Design review of the part shown in the three views and the two pictorial views. Dimensions are in mm from the part's minimum x, y and z. Give positions to 0.01 mm unless a question says otherwise; leave off trailing zeros. Order: outer loops, then holes, each group sorted by start corner. A loop starts at its lowest first (then second) coordinate and runs counter-clockwise, first axis right, second up.
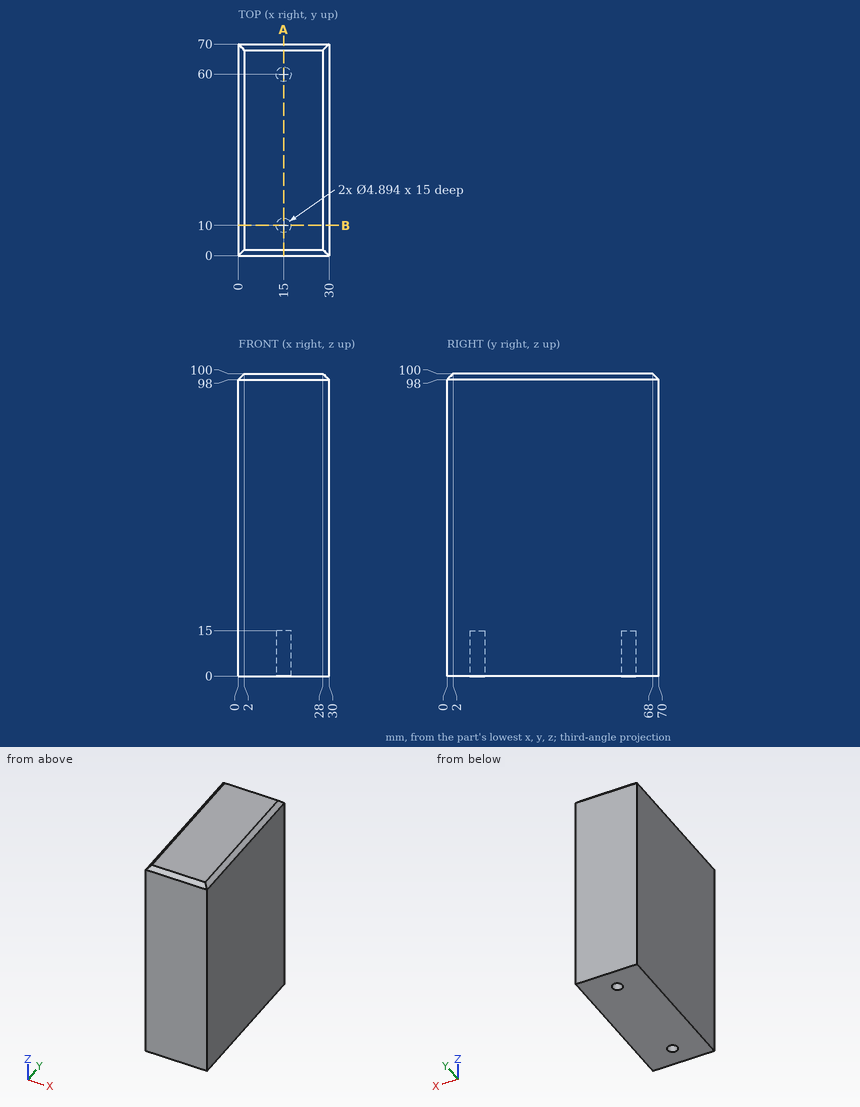
Item 1: For line 1 (Y direction, x = 15, z = 10); line 2 (X direction, y = 10, z = 7.25), list the stretches that pass through material, from the lowest coordinate up.
Values found:
line 1: y = 0 to 7.55, 12.45 to 57.55, 62.45 to 70
line 2: x = 0 to 12.55, 17.45 to 30
Item 2: Take a section at B-B (y = 10). Give the boundary of the cut face in (x, z), and give its area (3 significant figures).
Values found:
outline: (0, 0) - (12.55, 0) - (12.55, 15) - (17.45, 15) - (17.45, 0) - (30, 0) - (30, 98) - (28, 100) - (2, 100) - (0, 98) - close
area: 2,920 mm2
Item 3: Take a section at A-A (x = 15). Give the boundary of the cut face in (y, z).
Values found:
outline: (0, 0) - (7.55, 0) - (7.55, 15) - (12.45, 15) - (12.45, 0) - (57.55, 0) - (57.55, 15) - (62.45, 15) - (62.45, 0) - (70, 0) - (70, 98) - (68, 100) - (2, 100) - (0, 98) - close
Item 4: Clearance check with flat-ended pins moving along their axes: pin 1 Ø1 at (x, y) = (24, 61.5) entering from -Z; pin 2 Ø2.5 at (x, y) = (14.5, 9.5) entering from -Z. State where each tip first meets the part, or that it passes through.
Values found:
pin 1: stops at z = 0
pin 2: stops at z = 15
